```python
from build123d import *

# Parameters (mm, degrees)
SKETCH1_W                                       = 50
SKETCH1_H                                       = 20
BOSS_EXTRUDE1_DEPTH                             = 8
CSK_FOR_M6_FLAT_HEAD_MACHINE_SCREW1_D           = 6.6
CSK_FOR_M6_FLAT_HEAD_MACHINE_SCREW1_CSINK_D     = 12.6
CSK_FOR_M6_FLAT_HEAD_MACHINE_SCREW1_CSINK_ANGLE = 90
FILLET1_R                                       = 4
SKETCH3_W                                       = 12
SKETCH3_H                                       = 20
BOSS_EXTRUDE2_DEPTH                             = 60
BOSS_EXTRUDE3_DEPTH                             = 4


with BuildPart() as part:
    # Sketch1 → Boss-Extrude1 (new body)
    with BuildSketch(Plane(origin=(0, 0, 0), x_dir=(1, 0, 0), z_dir=(0, 1, 0))):
        Rectangle(SKETCH1_W, SKETCH1_H)
    extrude(amount=BOSS_EXTRUDE1_DEPTH)

    # CSK for M6 Flat Head Machine Screw1 (through all)
    with Locations(Plane(origin=(-15, 8, 0), x_dir=(0, 0, 1), z_dir=(0, 1, 0))):
        with Locations((0, 0), (0, 30)):
            CounterSinkHole(CSK_FOR_M6_FLAT_HEAD_MACHINE_SCREW1_D / 2, CSK_FOR_M6_FLAT_HEAD_MACHINE_SCREW1_CSINK_D / 2, counter_sink_angle=CSK_FOR_M6_FLAT_HEAD_MACHINE_SCREW1_CSINK_ANGLE)

    # Fillet1
    fillet1_edges = [part.edges().sort_by_distance(p)[0] for p in [
        (-25, 4, -10),
        (25, 4, -10),
        (25, 4, 10),
        (-25, 4, 10),
    ]]
    fillet(fillet1_edges, radius=FILLET1_R)

    # Sketch3 → Boss-Extrude2 (add)
    with BuildSketch(Plane(origin=(0, 8, 0), x_dir=(1, 0, 0), z_dir=(0, 1, 0))):
        Rectangle(SKETCH3_W, SKETCH3_H)
    extrude(amount=BOSS_EXTRUDE2_DEPTH)

    # Sketch4 → Boss-Extrude3 (add)
    with BuildSketch(Plane.XY):
        with BuildLine():
            Line((-6, 68), (-1.958548116, 75))
            Line((-1.958548116, 75), (1.5, 75))
            Line((1.5, 75), (1.5, 73))
            Line((1.5, 73), (0.8, 73))
            ThreePointArc((0.8, 73), (0, 72.2), (0.8, 71.4))
            Line((0.8, 71.4), (1.5, 71.4))
            Line((1.5, 71.4), (1.5, 68))
            Line((1.5, 68), (-6, 68))
        make_face()
    extrude(amount=BOSS_EXTRUDE3_DEPTH)


solid = part.part
```
The listing builds one solid part. Answer for the finished solid, in the listing's coordinates (mm). A direction names the side the tool comes from. Give positions to 0.01 mm unless a question says otherwise; leave off trailing zeros. Order: outer loops, then holes, each group sorted by start corner. A loop starts at its lowest first (then second) coordinate and runs counter-clockwise, first axis right, second up. Notation, with made-up numbers: (80, 48.5) -> (124, 48.5) arc R26 ccw to (124, 78.5) -> close; hole circle Ø5 at (-32.5, 14). An arc over 180 degrees is marked (long way). Write each question's results on one line, items separated by ' | '.
Q1. The part is cut by section B-B, the plane y = 27.5. Give the vertices of the cut face in (x, z).
Checked values:
outline: (-6, -10) -> (6, -10) -> (6, 10) -> (-6, 10) -> close
Q2. Which of the six approach directions +Z, -Z, +X, -X, +Y, -Y give full straight-line access (tool end or side, diameter ignored) to faces 1 (the face through (-1, 71, 4)), 2 (the face through (20, 8, -5)), 3 (the face through (-19.9, 8, 4.3)), 4 (the face through (-1, 71, 0))?
Checked values:
face 1: +Z, +X, -X, +Y | face 2: +Z, -Z, +X, +Y | face 3: +Z, -Z, -X, +Y | face 4: -Z, +X, -X, +Y
Q3. The part is cut by section A-A, the plane x = 4. Give the vertices of the cut face in (y, z), and give its area (3 significant figures).
Checked values:
outline: (0, -10) -> (68, -10) -> (68, 10) -> (0, 10) -> close | area: 1,360 mm^2
Q4. Each of these flat-tipped pins is pushed along its axis until it touches: P1, Ø3.5, axis at x = -4, y = 70.5, coming from the -Z side; P2, Ø10, axis at y = 30.5, z = -3.5, coming from the +X side; P3, Ø1.5, axis at x = 19.5, z = -2.5, coming from the +Y side; P4, Ø4, axis at x = -15, z = 0, coming from the +Y side. Where does it stop, or does it pass through?
Checked values:
P1: stops at z = 0 | P2: stops at x = 6 | P3: stops at y = 7.6 | P4: passes through
Q5. The part is cut by section D-D, the plane z = 7.5. Give the vertices of the cut face in (x, y).
Checked values:
outline: (-24.71, 0) -> (24.71, 0) -> (24.71, 8) -> (6, 8) -> (6, 68) -> (-6, 68) -> (-6, 8) -> (-24.71, 8) -> close
Q6. Straight lines are drawn through the part: probe 1 along X at (y, z) = (3.35, 0); probe 2 along Z at (x, y) = (15, 2); probe 3 along X at (y, z) = (38, 3.25). For each, find the intervals that lie inside material, in ascending order. Write a range as from..to.
Checked values:
probe 1: x = -25..-18.3, -11.7..11.7, 18.3..25 | probe 2: z = -10..-3.3, 3.3..10 | probe 3: x = -6..6
Q7. The part is cut by section C-C, the plane z = 1.5. State how many separate pieces and enclosed holes the cut face has, and give its area (3 significant figures).
Checked values:
separate pieces: 3 | enclosed holes: 0 | area: 1,040 mm^2
